Can you work these out from the model? Positions are in its coordinate system, mm. Face numbers are marked on the shaded views. Round coordinates to 2 decimals unless told otherwise and drop trailing zeros. Loops run counter-clockwise (first coordinate to the right, second up) from the corner with the lowest first, then second, coordinate; pieces in that order, holes last.
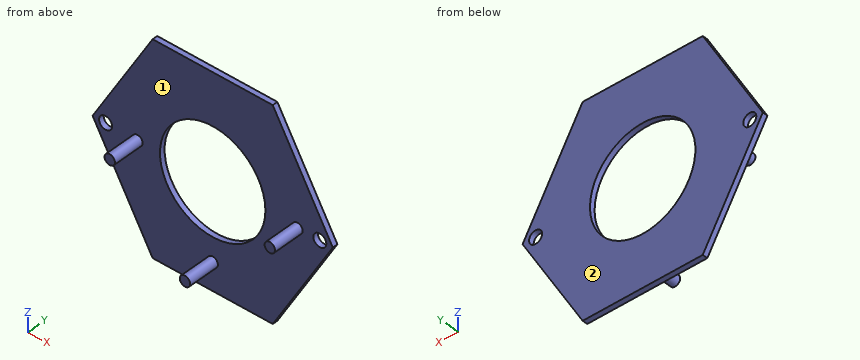
from build123d import *

# Parameters (mm, degrees)
BOSS_EXTRUDE1_DEPTH = 1
SKETCH3_R           = 1
BOSS_EXTRUDE2_DEPTH = 6
SKETCH4_R           = 10.135267165
CUT_EXTRUDE1_DEPTH  = 6
SKETCH5_R           = 1.25
CUT_EXTRUDE2_DEPTH  = 15


with BuildPart() as part:
    # Sketch1 → Boss-Extrude1 (new body)
    with BuildSketch(Plane(origin=(0, 0, 0), x_dir=(1, 0, 0), z_dir=(0, 1, 0))):
        Polygon((23.094010768, 0), (11.547005384, 20), (-11.547005384, 20), (-23.094010768, 0), (-11.547005384, -20), (11.547005384, -20), align=None)
    extrude(amount=BOSS_EXTRUDE1_DEPTH)

    # Sketch3 → Boss-Extrude2 (add)
    with BuildSketch(Plane.XZ):
        with Locations((16.308163565, 0)):
            Circle(SKETCH3_R)
        with Locations((-14.462214845, 0)):
            Circle(SKETCH3_R)
        with Locations((0, -14.675000966)):
            Circle(SKETCH3_R)
    extrude(amount=BOSS_EXTRUDE2_DEPTH)

    # Sketch4 → Cut-Extrude1 (cut)
    with BuildSketch(Plane(origin=(0, 1, 0), x_dir=(1, 0, 0), z_dir=(0, 1, 0))):
        Circle(SKETCH4_R)
    extrude(amount=-CUT_EXTRUDE1_DEPTH, mode=Mode.SUBTRACT)

    # Sketch5 → Cut-Extrude2 (cut)
    with BuildSketch(Plane(origin=(19.371137685, 1, -19.368583248), x_dir=(-1, 0, 0), z_dir=(0, 1, 0))):
        with Locations((-1.222873082, 19.368583248)):
            Circle(SKETCH5_R)
        with Locations((39.965148453, 19.368583248)):
            Circle(SKETCH5_R)
    extrude(amount=-CUT_EXTRUDE2_DEPTH, mode=Mode.SUBTRACT)


solid = part.part
(1) If we section it at D-D, the plane x = 16: List the corners of the cut face in (y, z) for me, then the cut area to 3 significant figures.
Worked answers:
outline: (-6, -0.95) - (0, -0.95) - (0, -12.29) - (1, -12.29) - (1, 12.29) - (0, 12.29) - (0, 0.95) - (-6, 0.95) - close
area: 36.0 mm2
(2) If we mould it in two halves opening along Y, with no side actions, what happens to the marked faces 1 and 2? For each: released by +Y, released by -Y, zero draft, split by the parting line, or undercut.
Worked answers:
face 1: released by -Y
face 2: released by +Y
(3) If we section it at C-C, the plane y = -3: List the corners of the cut face in (x, z) for me (3 decimals).
Worked answers:
outline: circle Ø2 at (-14.462, 0); circle Ø2 at (0, -14.675); circle Ø2 at (16.308, 0)
(4) Will these pins go through, and if not, where does the flat tip stop? P1, Ø3, axis at x = 20.59, z = 0, coming from the -Y side; P2, Ø1.5, axis at y = 0, z = 13, coming from the -X side; P3, Ø3, axis at x = -20.59, z = 0, coming from the +Y side; P4, Ø3, axis at x = 13.5, y = -2, coming from the +Z side.
Worked answers:
P1: stops at y = 0
P2: stops at x = -16.02
P3: stops at y = 1
P4: passes through
(5) If we section it at B-B, the plane z = -5: List the corners of the cut face in (x, y) for me.
Worked answers:
outline: (-20.21, 0) - (-8.82, 0) - (-8.82, 1) - (-20.21, 1) - close; (8.82, 0) - (20.21, 0) - (20.21, 1) - (8.82, 1) - close
(6) If we section it at A-A, the plane x = 0: List the corners of the cut face in (y, z) for me (3 decimals), then the cut area to 3 significant figures.
Worked answers:
outline: (-6, -15.675) - (0, -15.675) - (0, -20) - (1, -20) - (1, -10.135) - (0, -10.135) - (0, -13.675) - (-6, -13.675) - close; (0, 10.135) - (1, 10.135) - (1, 20) - (0, 20) - close
area: 31.7 mm2
(7) If I drill on line 1 (Z direction, x = 0, y = 0.6); line 2 (Y direction, x = 13, z = -10); line 3 (X direction, y = -3.25, z = -0.5), over which ranges is the centre line in solid material (lowest first)?
Worked answers:
line 1: z = -20 to -10.14, 10.14 to 20
line 2: y = 0 to 1
line 3: x = -15.33 to -13.6, 15.44 to 17.17
